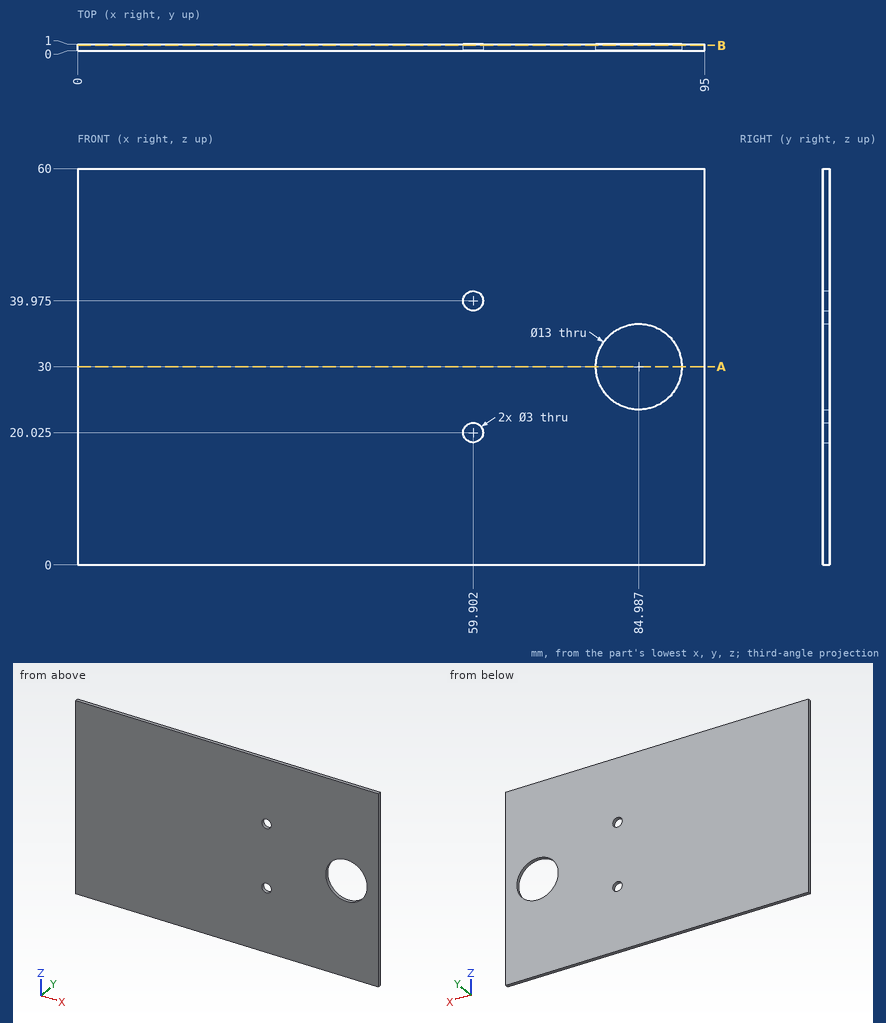
Study the drawing (mm; zero at the part's minimum x, y, z) and answer. Round coordinates to 2 decimals unless told otherwise and drop trailing zeros. Loops run counter-clockwise (first coordinate to the right, second up) from the corner with the lowest first, then second, coordinate; pieces in that order, holes last. Notation, with made-up numbers: (-33.5, 28) -> (-2.5, 28) arc R14 cw to (-2.5, 54) -> close; hole circle Ø5 at (22, -36.75). An arc over 180 degrees is marked (long way). Use one line per item in the form item = value.
1. A flat-ended cylindrical pin translates along its axis: pin 1 Ø3 at (x, z) = (12.5, 6.5) entering from -Y. Find the tip coordinate at first contact, or state that the pin passes through.
Answer key:
pin_1 = 0
2. Find the intervals of material crossed by probe 1 along X at (y, z) = (0.25, 30); probe 2 along X at (y, z) = (0.15, 20); probe 3 along Z at (x, y) = (60.5, 0.95), in increasing order. Write a range as [from, to].
Answer key:
probe_1 = [0, 78.49], [91.49, 95]
probe_2 = [0, 58.4], [61.4, 95]
probe_3 = [0, 18.65], [21.4, 38.6], [41.35, 60]
3. The part is cut by section B-B on y = 0.8. Determine the outline of the cut face in (x, z) (1 decimal).
Answer key:
outline = (0, 0) -> (95, 0) -> (95, 60) -> (0, 60) -> close; hole circle Ø3 at (59.9, 20); hole circle Ø3 at (59.9, 40); hole circle Ø13 at (85, 30)
4. The part is cut by section A-A on z = 30. Determine the outline of the cut face in (x, y).
Answer key:
outline = (0, 0) -> (78.49, 0) -> (78.49, 1) -> (0, 1) -> close; (91.49, 0) -> (95, 0) -> (95, 1) -> (91.49, 1) -> close
